Work out the finished part from the listing and answer in its coordinate system (mm). Face numbers are marked on the shaded views. A direction names the side the tool comes from. Coordinates: 2 decimals unless noted, no trailing zeros. Loops run counter-clockwise (first coordinate to the right, second up) from the corner with the lowest first, then second, coordinate; pieces in that order, holes last. Notation, with made-up numbers: (58, 80) -> (76, 80) arc R14 cw to (76, 85) -> close; hole circle Ø3 at (5.25, -36.5). An arc over 180 degrees is marked (long way). Use a Markdown table: item, result.
from build123d import *

# Parameters (mm, degrees)
F0_R     = 5
F1_DEPTH = 6
F2_R     = 3
F3_DEPTH = 26
F4_R     = 2.5
F5_DEPTH = 24
F7_DEPTH = 3
F8_SIZE  = 0.5


with BuildPart() as f1:
    # F0 (on Front) → F1 (new body)
    with BuildSketch(Plane.XZ):
        Circle(F0_R)
    extrude(amount=F1_DEPTH)

    # F2 (on face) → F3 (join)
    with BuildSketch(Plane(origin=(0, 0, 0), x_dir=(-1, 0, 0), z_dir=(0, 1, 0))):
        Circle(F2_R)
    extrude(amount=F3_DEPTH)

    # F4 (on face) → F5 (join)
    with BuildSketch(Plane(origin=(0, 26, 0), x_dir=(-1, 0, 0), z_dir=(0, 1, 0))):
        Circle(F4_R)
    extrude(amount=F5_DEPTH)

    # F6 (on face) → F7 (cut)
    with BuildSketch(Plane.XZ.offset(6)):
        Polygon((1.443376, 2.5), (-1.443376, 2.5), (-2.886751, 0), (-1.443376, -2.5), (1.443376, -2.5), (2.886751, 0), align=None)
    extrude(amount=-F7_DEPTH, mode=Mode.SUBTRACT)

    # F8
    f8_edges = [f1.edges().sort_by_distance(p)[0] for p in [
        (-5, -6, 0),
    ]]
    chamfer(f8_edges, length=F8_SIZE)


solid = f1.part
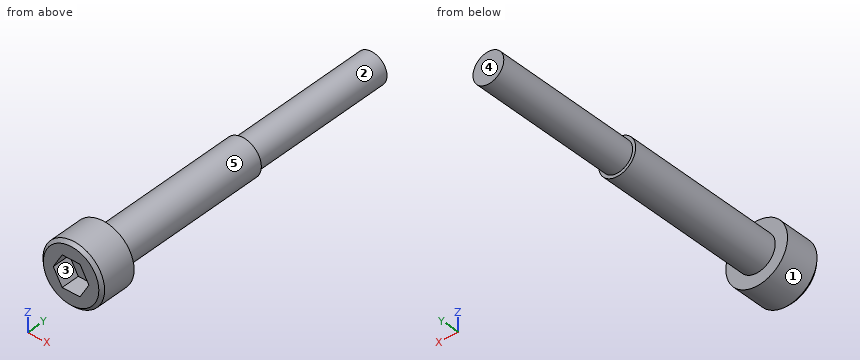
Q1. Determine the mould class of the marked faces 3, 4 and 5 for opening direction X: pulls with the +X half, pulls with the -X half, needs draft (parallel to the pull), parting line crosses it, or undercut.
Solved:
| item | result |
|---|---|
| face 3 | undercut |
| face 4 | needs draft |
| face 5 | parting line crosses it |
Q2. For the marked faces 1 and 2, determine the directions among +Z, -Z, +X, -X, +Y, -Y from which every point of the face is accessible in a straight line to the end or side of a thin tool.
Solved:
| item | result |
|---|---|
| face 1 | +Y, -Y |
| face 2 | +Y |
Q3. Consider line 1 (Y direction, x = -2.5, z = -0.75); line 2 (Y direction, x = 1.25, z = -3.5); line 3 (X direction, y = 30.5, z = -2). Determine where each line is inside the solid, lowest interval first. Write a range as [from, to].
Solved:
| item | result |
|---|---|
| line 1 | [-6, 26] |
| line 2 | [-6, 0] |
| line 3 | [-1.5, 1.5] |
Q4. Section C-C on y = 12.5 is taken. Determine the outline of the cut face in (x, z), and give its area (3 significant figures).
Solved:
| item | result |
|---|---|
| outline | circle Ø6 at (0, 0) |
| area | 28.3 mm² |
Q5. Section B-B on y = 32 is taken. Determine the outline of the cut face in (x, z).
Solved:
| item | result |
|---|---|
| outline | circle Ø5 at (0, 0) |
Q6. Section A-A on x = 0 is taken. Determine the outline of the cut face in (y, z).
Solved:
| item | result |
|---|---|
| outline | (-6, -4.5) -> (-5.5, -5) -> (0, -5) -> (0, -3) -> (26, -3) -> (26, -2.5) -> (50, -2.5) -> (50, 2.5) -> (26, 2.5) -> (26, 3) -> (0, 3) -> (0, 5) -> (-5.5, 5) -> (-6, 4.5) -> (-6, 2.5) -> (-3, 2.5) -> (-3, -2.5) -> (-6, -2.5) -> close |
Q7. Given pin 1 Ø4 at (y, z) = (40.5, -3.5) entering from -X; pin 2 Ø1.5 at (x, z) = (1.5, 3.5) entering from +Y, each flat-ended and moving along its own axis, determine where each tip first touches the part or whether it passes through.
Solved:
| item | result |
|---|---|
| pin 1 | x = -2 |
| pin 2 | y = 0 |
